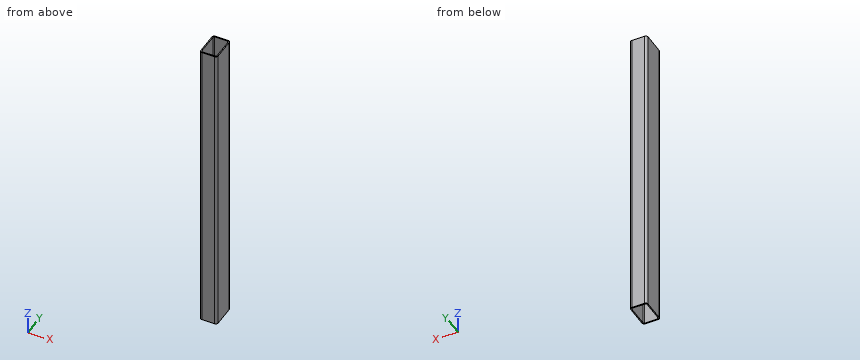
```python
from build123d import *

# Parameters (mm, degrees)
CNC_3X2X0_125_1_DEPTH = 900


with BuildPart() as part:
    # Sketch11 → Cnc 3X2X0.125(1) (new body)
    with BuildSketch(Plane.YX.offset(-450)):
        with BuildLine():
            Line((31.75, -25.4), (-31.75, -25.4))
            ThreePointArc((-31.75, -25.4), (-36.240128061, -23.540128061), (-38.1, -19.05))
            Line((-38.1, -19.05), (-38.1, 19.05))
            ThreePointArc((-38.1, 19.05), (-36.240128061, 23.540128061), (-31.75, 25.4))
            Line((-31.75, 25.4), (31.75, 25.4))
            ThreePointArc((31.75, 25.4), (36.240128061, 23.540128061), (38.1, 19.05))
            Line((38.1, 19.05), (38.1, -19.05))
            ThreePointArc((38.1, -19.05), (36.240128061, -23.540128061), (31.75, -25.4))
        make_face()
        with BuildLine():
            Line((31.75, 22.225), (-31.75, 22.225))
            ThreePointArc((-31.75, 22.225), (-33.99506403, 21.29506403), (-34.925, 19.05))
            Line((-34.925, 19.05), (-34.925, -19.05))
            ThreePointArc((-34.925, -19.05), (-33.99506403, -21.29506403), (-31.75, -22.225))
            Line((-31.75, -22.225), (31.75, -22.225))
            ThreePointArc((31.75, -22.225), (33.99506403, -21.29506403), (34.925, -19.05))
            Line((34.925, -19.05), (34.925, 19.05))
            ThreePointArc((34.925, 19.05), (33.99506403, 21.29506403), (31.75, 22.225))
        make_face(mode=Mode.SUBTRACT)
    extrude(amount=CNC_3X2X0_125_1_DEPTH)


solid = part.part
```
Model file for the job. Use its own axes, mm. Give positions to 0.01 mm unless a question says otherwise; leave off trailing zeros. Write each loop counter-clockwise with the first axis right and the second up, starting at its lowest first coordinate (ties: lowest second). Pieces come first, ordered by that corner, then holes. Notation, with made-up numbers: M 19,88 L 40,88 A16 cw 40,118 Z; hole C 50.5,20.25 d6. An arc over 180 degrees is marked long. Use a Markdown table: item, result.
1) Cut at B-B (x = -2). List the corners of the cut face in (y, z) (3 decimals).
Responses:
| item | result |
|---|---|
| outline | M -38.1,-450 L -34.925,-450 L -34.925,450 L -38.1,450 Z; M 34.925,-450 L 38.1,-450 L 38.1,450 L 34.925,450 Z |
2) Cut at C-C (z = -287.5). List the corners of the cut face in (x, y) (3 decimals), and give its area (3 significant figures).
Responses:
| item | result |
|---|---|
| outline | M -25.4,-31.75 A6.35 ccw -19.05,-38.1 L 19.05,-38.1 A6.35 ccw 25.4,-31.75 L 25.4,31.75 A6.35 ccw 19.05,38.1 L -19.05,38.1 A6.35 ccw -25.4,31.75 Z; hole M -22.225,-31.75 A3.175 ccw -19.05,-34.925 L 19.05,-34.925 A3.175 ccw 22.225,-31.75 L 22.225,31.75 A3.175 ccw 19.05,34.925 L -19.05,34.925 A3.175 ccw -22.225,31.75 Z |
| area | 740 mm2 |
3) Cut at A-A (y = -4). List the corners of the cut face in (x, z) (3 decimals).
Responses:
| item | result |
|---|---|
| outline | M -25.4,-450 L -22.225,-450 L -22.225,450 L -25.4,450 Z; M 22.225,-450 L 25.4,-450 L 25.4,450 L 22.225,450 Z |
4) Pin check, flat tip, straight feed: pin 1 (10 mm diameter, centred on x = 14, y = 15.5, fed in from +Z). Stop position of the tip, or through.
Responses:
| item | result |
|---|---|
| pin 1 | passes through |
5) Drill centre lines: line 1 (X direction, y = -9, z = 26.5) (3 decimals); line 2 (Y direction, x = -1, z = 2.5) (3 decimals); line 3 (X direction, y = -34, z = 63.5). Where is each one in solid material? Low to high. Write a range as from..to.
Responses:
| item | result |
|---|---|
| line 1 | x = -25.4..-22.225, 22.225..25.4 |
| line 2 | y = -38.1..-34.925, 34.925..38.1 |
| line 3 | x = -24.99..-21.29, 21.29..24.99 |
